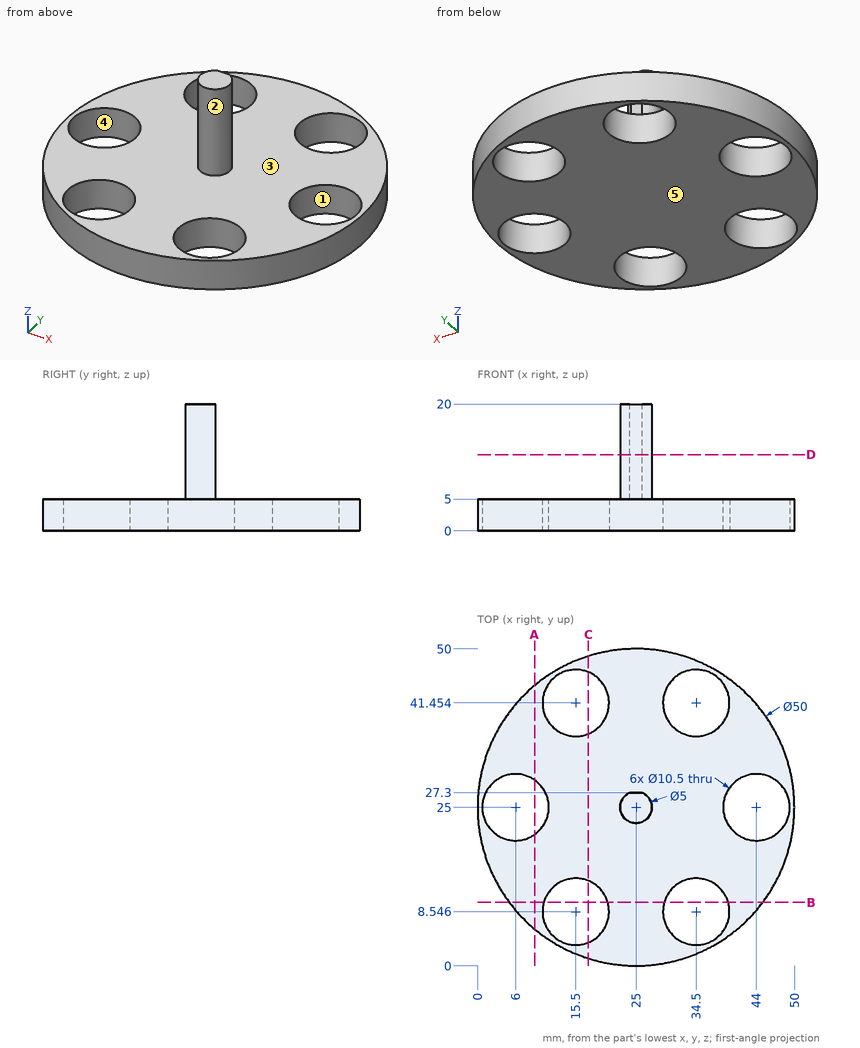
Design review of the part shown in the three views and the two pictorial views. Dimensions are in mm from the part's minimum x, y and z. A direction names the side the tool comes from. Round coordinates to 2 decimals unless told otherwise and drop trailing zeros. Write each loop counter-clockwise with the first axis right and the second up, starting at its lowest first coordinate (ties: lowest second). Pieces come first, ordered by that corner, then holes. Notation, with made-up numbers: (69, 75) - (74, 75) arc R27 cw to (74, 109) - close; hole circle Ø10 at (-26.5, 7.25). An arc over 180 degrees is marked (long way). Write item = value, one per line. Start each with the question number.
1. Consider section A-A on x = 9. State the section outline as (y, z) points.
2. For the marked faces 1 and 2, list the 3-axis set-ups (+Z, -Z, +X, -X, +Y, -Y) from which the entire face can be reached by the end or side of a thin tool; tool diameter is ignored.
3. Draft analysis for pull direction Z (two halves, no side actions). For the marked faces 3, 4 and 5, state which applies: released by +Z, released by -Z, zero draft, split by the parting line, or undercut.
4. Consider section C-C on x = 17.5. State the section outline as (y, z) points.
5. For pin 1 Ø10 at (x, z) = (26.5, 9) entering from +Y; pin 2 Ø5 at (x, y) = (36.5, 41.5) entering from +Z; pin 3 Ø1 at (x, z) = (24.5, 16) entering from +Y; pin 4 Ø12 at (x, y) = (44, 23) entering from +Z, all flat-tipped, find the tip position at first contact; note any pin that passes through.
6. Consider section B-B on y = 10. State the section outline as (x, z) points (1 decimal).
7. Consider section D-D on z = 12. State the section outline as (x, y) points, plus the area to 3 significant figures.
8. Wall thickness on L1, parallel to Y at x = 15.5, z = 3.55 (1 decimal); L2, parallel to X at y = 27.5, z = 4.25 (1 decimal); L3, parallel to Z at x = 37.5, y = 13: over which ranges is each line inside the solid? List them lowest first.
Evaluation:
q1.outline = (5.79, 0) - (20.69, 0) - (20.69, 5) - (5.79, 5) - close; (29.31, 0) - (44.21, 0) - (44.21, 5) - (29.31, 5) - close
q2.face_1 = +Z, -Z
q2.face_2 = +Z
q3.face_3 = released by +Z
q3.face_4 = zero draft
q3.face_5 = released by -Z
q4.outline = (1.15, 0) - (3.69, 0) - (3.69, 5) - (1.15, 5) - close; (13.4, 0) - (36.6, 0) - (36.6, 5) - (13.4, 5) - close; (46.31, 0) - (48.85, 0) - (48.85, 5) - (46.31, 5) - close
q5.pin_1 = 50
q5.pin_2 = through
q5.pin_3 = 27.3
q5.pin_4 = 5
q6.outline = (5, 0) - (10.5, 0) - (10.5, 5) - (5, 5) - close; (20.5, 0) - (29.5, 0) - (29.5, 5) - (20.5, 5) - close; (39.5, 0) - (45, 0) - (45, 5) - (39.5, 5) - close
q7.outline = (24.02, 27.3) arc R2.5 ccw (long way) to (25.98, 27.3) - close
q7.area = 19.4 mm2
q8.L1 = 1.9 to 3.3, 13.8 to 36.2, 46.7 to 48.1
q8.L2 = 0.1 to 1.4, 10.6 to 39.4, 48.6 to 49.9
q8.L3 = 0 to 5
